Geometry check sheet. Reference: the model listing, model coordinates, mm. A direction names the side the tool comes from. Coordinates: 2 decimals unless noted, no trailing zeros. Write each loop counter-clockwise with the first axis right and the second up, starting at its lowest first coordinate (ties: lowest second). Pieces come first, ordered by that corner, then holes. Notation, with made-up numbers: M 32,35 L 65,35 A22 cw 65,72 Z; hole C 75,19 d8. An arc over 180 degrees is marked long. Put each result on its own line as item: value. Start each with the question number.
1) Set-up check for faces 1 (the cylindrical face through (77.389, -4.736, 50.527)), 2 (the cylindrical face through (39.45, -40.2, 20.85)), 3 (the cylindrical face through (4.491, -122.264, 11.02)), 4 (the cylindrical face through (77.389, -122.264, 50.527)), 5 (the flat face through (142, 0, 40)): record each of +Z, -Z, +X, -X, +Y, -Y from which the full face is reachable in a straight line by a thin tool's end or side.
2) Gauge pin test, flat ends, axial feed: pin 1 (12 mm diameter, centred on x = 65.5, y = -85.5, fed in from +Z); pin 2 (8.5 mm diameter, centred on x = 152.4, y = -31.75, fed in from +Z); pin 3 (5.5 mm diameter, centred on x = 36, y = -30, fed in from +Z). Record the tip position at first contact, or that the pin passes through.
3) Mould release check, pull along Y, two halves, no side actions. Record for faces 6 (the flat face through (142, -127, 40)), 7 (the flat face through (158, -63, 79.502)), 8 (the flat face through (33, -29, 19.304)), 9 (the flat face through (150, -29, 73.152)): released by +Y, released by -Y, zero draft, split by the parting line, or undercut.
4) Cross-section at C-C on z = 58. Record the cut outline in (x, y) (3 decimals), plus the area to 3 significant figures.
5) Scan lines: line 1 along Y through (x, z) = (114, 76); line 2 along X through (y, z) = (-31, 75); line 3 along Y through (x, z) = (152, 50). Record each from-to range of solid material in increasing order.
6) Cross-section at A-A on z = 31.5. Record the cut outline in (x, y), plus the area to 3 significant figures.
7) Cross-section at B-B on x = 76. Record the cut outline in (y, z).
from build123d import *

# Parameters (mm, degrees)
F1_DEPTH       = 127
F2_R           = 15.748
F4_D           = 6.35
F4_DEPTH       = 38.1
F4_CBORE_D     = 19.05
F4_CBORE_DEPTH = 6.35
F4_TIP         = 1.9077324654
F5_D           = 6.35
F5_DEPTH       = 3.048
F5_START       = 57.15
F5_CBORE_D     = 19.05
F5_CBORE_DEPTH = 3.048
F5_TIP         = 1.9077324654


with BuildPart() as f1:
    # F0 (on Front) → F1 (new body)
    with BuildSketch(Plane.XZ):
        Polygon((0, 22.352), (0, 0), (241.3, 0), (241.3, 79.502), (72.898, 79.502), (72.898, 22.352), align=None)
    extrude(amount=F1_DEPTH)

    # F2
    f2_edges = [f1.edges().sort_by_distance(p)[0] for p in [
        (0, -127, 11.176),
        (0, 0, 11.176),
        (72.898, -127, 50.927),
        (72.898, 0, 50.927),
        (241.3, -127, 39.751),
        (241.3, 0, 39.751),
    ]]
    fillet(f2_edges, radius=F2_R)

    # F4
    with Locations(Plane.XY.offset(79.502)):
        with Locations((152.4, -31.75), (114.3, -91.948)):
            CounterBoreHole(F4_D / 2, F4_CBORE_D / 2, F4_CBORE_DEPTH, depth=F4_DEPTH)
            with Locations((0, 0, -(F4_DEPTH + F4_TIP / 2))):  # 118° drill point
                Cone(0, F4_D / 2, F4_TIP, mode=Mode.SUBTRACT)

    # F5
    # its depths count from where the whole tool has entered the part; down to there all is cleared
    with Locations(Plane.XY.offset(79.502)):
        with Locations((35.052, -31.75)):
            Hole(F5_CBORE_D / 2, depth=F5_START)
    with Locations(Plane.XY.offset(79.502)):
        with Locations((199.898, -91.948, 0), (35.052, -31.75, -F5_START)):
            CounterBoreHole(F5_D / 2, F5_CBORE_D / 2, F5_CBORE_DEPTH, depth=F5_DEPTH)
            with Locations((0, 0, -(F5_DEPTH + F5_TIP / 2))):  # 118° drill point
                Cone(0, F5_D / 2, F5_TIP, mode=Mode.SUBTRACT)


solid = f1.part
Answer key:
1. face 1: +Z, -X, +Y
1. face 2: +Z
1. face 3: +Z, -Z, -X, -Y
1. face 4: +Z, -X, -Y
1. face 5: +Z, -Z, +X, -X, +Y
2. pin 1: stops at z = 22.35
2. pin 2: stops at z = 73.15
2. pin 3: stops at z = 19.3
3. face 6: released by -Y
3. face 7: zero draft
3. face 8: undercut
3. face 9: undercut
4. outline: M 72.898,-111.252 A15.748 ccw 88.646,-127 L 225.552,-127 A15.748 ccw 241.3,-111.252 L 241.3,-15.748 A15.748 ccw 225.552,0 L 88.646,0 A15.748 ccw 72.898,-15.748 Z; hole C 114.3,-91.948 d6.35; hole C 152.4,-31.75 d6.35
4. area: 21,100 mm²
5. line 1: y = -127 to -101.47, -82.43 to 0
5. line 2: x = 72.9 to 142.9, 161.9 to 241.3
5. line 3: y = -127 to -34.9, -28.6 to 0
6. outline: M 72.9,-111.25 A15.75 ccw 88.65,-127 L 225.55,-127 A15.75 ccw 241.3,-111.25 L 241.3,-15.75 A15.75 ccw 225.55,0 L 88.65,0 A15.75 ccw 72.9,-15.75 Z
6. area: 21,200 mm²
7. outline: M -127,0 L 0,0 L 0,22.35 L -6.36,22.35 L -6.36,79.5 L -120.64,79.5 L -120.64,22.35 L -127,22.35 Z
